from build123d import *

# Parameters (mm, degrees)
F0_W     = 192.7
F0_H     = 112.7
F1_DEPTH = 6.35
F2_W     = 96.7
F2_H     = 96.7
F2_W_2   = 5
F2_H_2   = 65
F3_DEPTH = 6.351


with BuildPart() as f1:
    # F0 (on Top) → F1 (new body)
    with BuildSketch(Plane.XY):
        Rectangle(F0_W, F0_H)
    extrude(amount=F1_DEPTH)

    # F2 (on face) → F3 (cut, through all)
    with BuildSketch(Plane.XY.offset(6.35)):
        Rectangle(F2_W, F2_H)
        with Locations((-59.85, 0)):
            Rectangle(F2_W_2, F2_H_2)
        with Locations((59.85, 0)):
            Rectangle(F2_W_2, F2_H_2)
    extrude(amount=-F3_DEPTH, mode=Mode.SUBTRACT)


solid = f1.part
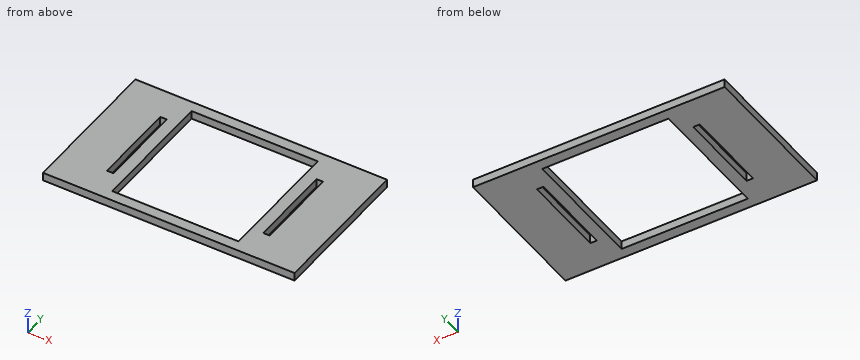
For this review, take the finished solid that the model builds, in its own axes (mm). Coordinates: 2 decimals unless noted, no trailing zeros. Loops run counter-clockwise (first coordinate to the right, second up) from the corner with the lowest first, then second, coordinate; pieces in that order, holes last. Notation, with made-up numbers: (10.5, 61.5) - (45.5, 61.5) arc R34 cw to (45.5, 100.5) - close; hole circle Ø11 at (-6.75, 88). An arc over 180 degrees is marked (long way). Use a Markdown table: item, result. Add a question column.
Item 1: For line 1 (X direction, y = -11, z = 6); line 2 (Y direction, x = 10.5, z = 3); line 3 (X direction, y = -43, z = 4.5), list the stretches that pass through material, from the lowest coordinate up.
Item 2: We need section B-B (y = -16). Give the boundary of the cut face in (x, z).
Item 3: We need section A-A (z = 4). Give the boundary of the cut face in (x, y).
Item 4: We need section C-C (x = 60.5). Give the boundary of the cut face in (y, z), and give its area (3 significant figures).
Item 5: We need section D-D (y = -38.5). Give the boundary of the cut face in (x, z), and give its area (3 significant figures).
Results list:
| question | item | result |
|---|---|---|
| 1 | line 1 | x = -96.35 to -62.35, -57.35 to -48.35, 48.35 to 57.35, 62.35 to 96.35 |
| 1 | line 2 | y = -56.35 to -48.35, 48.35 to 56.35 |
| 1 | line 3 | x = -96.35 to -48.35, 48.35 to 96.35 |
| 2 | outline | (-96.35, 0) - (-62.35, 0) - (-62.35, 6.35) - (-96.35, 6.35) - close; (-57.35, 0) - (-48.35, 0) - (-48.35, 6.35) - (-57.35, 6.35) - close; (48.35, 0) - (57.35, 0) - (57.35, 6.35) - (48.35, 6.35) - close; (62.35, 0) - (96.35, 0) - (96.35, 6.35) - (62.35, 6.35) - close |
| 3 | outline | (-96.35, -56.35) - (96.35, -56.35) - (96.35, 56.35) - (-96.35, 56.35) - close; hole (-62.35, -32.5) - (-57.35, -32.5) - (-57.35, 32.5) - (-62.35, 32.5) - close; hole (-48.35, -48.35) - (48.35, -48.35) - (48.35, 48.35) - (-48.35, 48.35) - close; hole (57.35, -32.5) - (62.35, -32.5) - (62.35, 32.5) - (57.35, 32.5) - close |
| 4 | outline | (-56.35, 0) - (-32.5, 0) - (-32.5, 6.35) - (-56.35, 6.35) - close; (32.5, 0) - (56.35, 0) - (56.35, 6.35) - (32.5, 6.35) - close |
| 4 | area | 303 mm^2 |
| 5 | outline | (-96.35, 0) - (-48.35, 0) - (-48.35, 6.35) - (-96.35, 6.35) - close; (48.35, 0) - (96.35, 0) - (96.35, 6.35) - (48.35, 6.35) - close |
| 5 | area | 610 mm^2 |
